from build123d import *

# Parameters (mm, degrees)
SKETCH1_R               = 35
SKETCH1_R_2             = 25
SKETCH1_R_3             = 20
BOSS_EXTRUDE1_DEPTH     = 10
BOSS_EXTRUDE4_START     = -300
SKETCH1_6_R             = 25
SKETCH1_6_R_2           = 20
BOSS_EXTRUDE4_DEPTH     = 300
CUT_EXTRUDE2_DEPTH      = 305.05591591
CUT_EXTRUDE2_DEPTH_BACK = 305.05591591
SKETCH2_R               = 7.5


with BuildPart() as part:
    # Sketch1 → Boss-Extrude1 (new body)
    # profile 1 of 2: a face of its own
    with BuildSketch(Plane(origin=(0, 0, 0), x_dir=(1, 0, 0), z_dir=(0, 1, 0))):
        with Locations(Location((0, 0, 0), (0, 0, 270))):
            Circle(SKETCH1_R)
        Circle(SKETCH1_R_2, mode=Mode.SUBTRACT)
    # profile 2 of 2: a face of its own
    with BuildSketch(Plane(origin=(0, 0, 0), x_dir=(1, 0, 0), z_dir=(0, 1, 0))):
        Circle(SKETCH1_R_2)
        with Locations(Location((0, 0, 0), (0, 0, 270))):
            Circle(SKETCH1_R_3, mode=Mode.SUBTRACT)
    extrude(amount=BOSS_EXTRUDE1_DEPTH)

    # Sketch1_6 → Boss-Extrude4 (add)
    with BuildSketch(Plane(origin=(0, 0, 0), x_dir=(1, 0, 0), z_dir=(0, 1, 0)).offset(BOSS_EXTRUDE4_START)):
        with Locations(Location((0, 0, 0), (0, 0, 270))):
            Circle(SKETCH1_6_R)
        with Locations(Location((0, 0, 0), (0, 0, 270))):
            Circle(SKETCH1_6_R_2, mode=Mode.SUBTRACT)
    extrude(amount=BOSS_EXTRUDE4_DEPTH)

    # Sketch2 → Cut-Extrude2 (cut, two sides: drawn at the far end of the back side and taken through both)
    with BuildSketch(Plane(origin=(0, 0, 0), x_dir=(0, 0, -1), z_dir=(1, 0, 0)).offset(-CUT_EXTRUDE2_DEPTH_BACK)):
        with Locations((0, -280)):
            Circle(SKETCH2_R)
    extrude(amount=CUT_EXTRUDE2_DEPTH + CUT_EXTRUDE2_DEPTH_BACK, mode=Mode.SUBTRACT)


solid = part.part
For this review, take the finished solid that the model builds, in its own axes (mm). Coordinates: 2 decimals unless noted, no trailing zeros. Order: outer loops, then holes, each group sorted by start corner. A loop starts at its lowest first (then second) coordinate and runs counter-clockwise, first axis right, second up. Notation, with made-up numbers: (56.5, 60) - (92.5, 60) arc R17 ccw to (92.5, 78) - close; hole circle Ø11 at (9, 82.5). An arc over 180 degrees is marked (long way). Use one line per item in the form item = value.
Q1. For probe 1 along Y at (x, z) = (-20.5, 0); probe 2 along X at (y, z) = (-74, 0); probe 3 along Y at (x, z) = (23, 2), list the stretches that pass through material, from the lowest coordinate up. Write a range as from..to.
Checked values:
probe_1 = -300..-287.5, -272.5..10
probe_2 = -25..-20, 20..25
probe_3 = -300..-287.23, -272.77..10
Q2. Consider section A-A (x = 0). Give the boundary of the cut face in (y, z), then the cut area to 3 significant figures.
Checked values:
outline = (-300, -25) - (0, -25) - (0, -35) - (10, -35) - (10, -20) - (-300, -20) - close; (-300, 20) - (10, 20) - (10, 35) - (0, 35) - (0, 25) - (-300, 25) - close
area = 3,300 mm2
Q3. Consider section D-D (y = -175.5). Give the boundary of the cut face in (x, z), then the cut area to 3 significant figures.
Checked values:
outline = circle Ø50 at (0, 0); hole circle Ø40 at (0, 0)
area = 707 mm2
Q4. Draft analysis for pull direction X (two halves, no side actions). For faces 1 (the cylindrical face through (-22.2, -152.1, 11.5)), 2 (the cylindrical face through (6.007, -147.17, 19.076)), 3 (the flat face through (-24, 0, -8)), state which applies: +X half, -X half, draft (parallel to the pull), parting line (faces both ways), or undercut.
Checked values:
face_1 = parting line
face_2 = undercut
face_3 = draft
Q5. Consider section B-B (z = 0). Give the boundary of the cut face in (x, y).
Checked values:
outline = (-35, 0) - (-25, 0) - (-25, -272.5) - (-20, -272.5) - (-20, 10) - (-35, 10) - close; (-25, -300) - (-20, -300) - (-20, -287.5) - (-25, -287.5) - close; (20, -300) - (25, -300) - (25, -287.5) - (20, -287.5) - close; (20, -272.5) - (25, -272.5) - (25, 0) - (35, 0) - (35, 10) - (20, 10) - close
Q6. For P1, Ø4, axis at x = 5.5, y = -30, coming from the -Z side; P2, Ø1.5, axis at x = -21, y = -217.5, coming from the +Z side; P3, Ø10, axis at x = -13, y = -60, coming from the -Z side, all flat-tipped, find the tip position at first contact; note any pin that passes through.
Checked values:
P1 = -24.75
P2 = 14.66
P3 = -23.69
Q7. Consider section C-C (y = -280). Give the boundary of the cut face in (x, z), then the cut area to 3 significant figures.
Checked values:
outline = (-23.85, -7.5) arc R25 ccw to (23.85, -7.5) - (18.54, -7.5) arc R20 cw to (-18.54, -7.5) - close; (-23.85, 7.5) - (-18.54, 7.5) arc R20 cw to (18.54, 7.5) - (23.85, 7.5) arc R25 ccw to start
area = 554 mm2
